Geometry: final body of the model. Coordinates: model frame, mm. A direction names the side the tool comes from. Coordinates: 2 decimals unless noted, no trailing zeros. Write each loop counter-clockwise with the first axis right and the second up, starting at its lowest first coordinate (ties: lowest second). Pieces come first, ordered by that corner, then holes.
Autodesk Inventor part; units mm, degrees
ref_plane "YZ Plane" through (0, 0, 0) normal (1, 0, 0) x (0, 1, 0)
ref_plane "XZ Plane" through (0, 0, 0) normal (0, 1, 0) x (-1, 0, 0)
ref_plane "XY Plane" through (0, 0, 0) normal (0, 0, 1) x (1, 0, 0)
sketch "Sketch1" plane through (0, 0, 0) normal (0, 0, 1) x (1, 0, 0)
  circle A0 centre (19.05, 19.05) radius 7.9375
  line L0 (22.7162, 25.4) -> (26.3823, 19.05)
  line L1 (26.3823, 19.05) -> (22.7162, 12.7)
  line L2 (22.7162, 12.7) -> (15.3838, 12.7)
  line L3 (15.3838, 12.7) -> (11.7177, 19.05)
  line L4 (11.7177, 19.05) -> (15.3838, 25.4)
  line L5 (15.3838, 25.4) -> (22.7162, 25.4)
  circle A1 centre (0, 19.05) radius 2.0828
  line L6 (0, 19.05) -> (19.05, 19.05) construction
  circle A2 centre (9.525, 2.5522) radius 2.0828
  circle A3 centre (28.575, 2.5522) radius 2.0828
  circle A4 centre (38.1, 19.05) radius 2.0828
  circle A5 centre (28.575, 35.5478) radius 2.0828
  circle A6 centre (9.525, 35.5478) radius 2.0828
  circle A7 centre (19.05, 19.05) radius 25.4
  line L7 (19.05, -6.35) -> (-19.05, -6.35)
  line L8 (-19.05, -6.35) -> (-19.05, 57.15)
  line L9 (6.3948, 114.3) -> (92.075, 114.3)
  line L10 (92.075, 114.3) -> (92.075, 63.5)
  line L11 (92.075, 63.5) -> (29.3317, 63.5)
  line L12 (-121.3454, 55.7276) -> (199.3502, 55.7276) construction
  arc A8 (29.3317, 63.5) -> (26.369, 43.3727) centre (29.3317, 53.2183) ccw
  circle A9 centre (85.725, 69.85) radius 2.0828
  circle A10 centre (85.725, 82.55) radius 2.0828
  circle A11 centre (85.725, 95.25) radius 2.0828
  circle A12 centre (85.725, 107.95) radius 2.0828
  line L13 (29.3317, 53.2183) -> (19.05, 53.2183) construction
  line L14 (-19.05, 57.15) -> (6.3948, 114.3)
  circle A13 centre (-12.7, 47.625) radius 2.0828
  circle A14 centre (6.35, 47.625) radius 2.0828
  circle A15 centre (-12.7, 22.225) radius 2.0828
  circle A16 centre (12.7, 78.7335) radius 2.0828
  circle A17 centre (12.7, 100.9585) radius 2.0828
  point P0 (0, 0)
  point P1 (19.05, 44.45)
  dimension "d7" = 15.875
  dimension "d8" = 12.7
  dimension "d23" = 4.1656
  dimension "d25" = 19.05
  dimension "d26" = 0
  dimension "d29" = 360
  dimension "d41" = 50.8
  dimension "d42" = 19.05
  dimension "d43" = 19.05
  dimension "d44" = 38.1
  dimension "d55" = 73.025
  dimension "d57" = 4.1656
  dimension "d58" = 6.35
  dimension "d59" = 6.35
  dimension "d62" = 12.7
  dimension "d67" = 6.35
  dimension "d68" = 36.6776
  dimension "d69" = 50.8
  dimension "d70" = 38.1
  dimension "d71" = 114
  dimension "d72" = 57.15
  dimension "d76" = 56.3933
  dimension "d78" = 6.35
  dimension "d79" = 9.525
  dimension "d84" = 19.05
  dimension "d91" = 31.75
  dimension "d98" = 25.4
  dimension "d105" = 22.225
  dimension "d113" = 6.35
extrude "Extrusion1" add sketch "Sketch1" along normal blind 3.175 contours A0 | A7 | A7 L7 L8 L14 L9 L10 L11 A8
sketch "Sketch2" plane through (0, 0, 3.175) normal (0, 0, 1) x (1, 0, 0)
  line L0 (-19.05, -6.35) -> (19.05, -6.35)
  arc A0 (19.05, -6.35) -> (26.369, 43.3727) centre (19.05, 19.05) ccw
  line L1 (-19.05, 57.15) -> (-19.05, -6.35)
  circle A1 centre (19.05, 19.05) radius 25.4
  line L2 (2.1167, 0.118) -> (-19.05, 19.05)
  line L3 (-19.05, 19.05) -> (-19.05, -6.35)
  line L4 (-19.05, -6.35) -> (19.05, -6.35)
  arc A2 (2.1167, 0.118) -> (19.05, -6.35) centre (19.05, 19.05) ccw
  point P0 (-19.05, 56.4751)
  point P1 (0, 0)
  dimension "d110" = 25.4
extrude "Extrusion2" cut sketch "Sketch2" against normal blind 25.4 contours L1 L2 A1 L0
fillet "Fillet2" radius 3.175 5 edges at (6.3948, 114.3, 1.5875) (-19.05, 57.15, 1.5875) (-19.05, 19.05, 1.5875) (92.075, 63.5, 1.5875) (92.075, 114.3, 1.5875)
equation "\"d67\" = d58"
properties part number "Lexan flexible Arm Mount" material "Polycarbonate, Clear"
Item 1: Section C-C, the plane x = -12.7. Output: boundary loops of the cut face in (y, z) (3 decimals).
Derived:
outline: (13.37, 0) - (20.142, 0) - (20.142, 3.175) - (13.37, 3.175) - close; (24.308, 0) - (45.542, 0) - (45.542, 3.175) - (24.308, 3.175) - close; (49.708, 0) - (71.412, 0) - (71.412, 3.175) - (49.708, 3.175) - close
Item 2: Section A-A, the plane x = 42.5. Output: boundary loops of the cut face in (y, z) (3 decimals).
Derived:
outline: (9.29, 0) - (28.81, 0) - (28.81, 3.175) - (9.29, 3.175) - close; (63.5, 0) - (114.3, 0) - (114.3, 3.175) - (63.5, 3.175) - close
Item 3: Pull-direction query (X, two-part tool) for faces 4 (the flat face through (92.075, 89, 2)), 5 (the cylindrical face through (85.273, 97.283, 1.565)), 6 (the cylindrical face through (6.75, 113.8, 1.61)); classes: released by +X, released by -X, zero draft, split by the parting line, or undercut.
Derived:
face 4: released by +X
face 5: undercut
face 6: released by -X
Item 4: Section D-D, the plane z = 2.6. State how many separate pieces and enclosed holes the cut face has, plus the area to 3 significant figures.
Derived:
separate pieces: 1
enclosed holes: 16
area: 7,910 mm2
Item 5: Section B-B, the plane y = 82.55. Output: boundary loops of the cut face in (x, z) (3 decimals), plus the area to 3 significant figures.
Derived:
outline: (-7.741, 0) - (83.642, 0) - (83.642, 3.175) - (-7.741, 3.175) - close; (87.808, 0) - (92.075, 0) - (92.075, 3.175) - (87.808, 3.175) - close
area: 304 mm2
Item 6: Set-up query: faces 1 (the flat face through (19, 12.7, 2)), 2 (the flat face through (-7.797, 8.985, 1.61)), 3 (the flat face through (60, 63.5, 2)). Return all of +Z, -Z, +X, -X, +Y, -Y with unobstructed straight access to the full face (end or side cutting, diameter ignored); none if empty.
Derived:
face 1: +Z, -Z
face 2: +Z, -Z, -X, -Y
face 3: +Z, -Z, +X
Item 7: Material intervals for probe 1 along Y at (x, z) = (-12.7, 1.25); probe 2 along X at (y, z) = (49, 2); probe 3 along Y at (x, z) = (14.5, 2.4), sorted ascending.
Derived:
probe 1: y = 13.37 to 20.14, 24.31 to 45.54, 49.71 to 71.41
probe 2: x = -19.05 to -14.26, -11.14 to 4.79, 7.91 to 19.96
probe 3: y = -5.94 to 14.23, 23.87 to 77.69, 79.78 to 99.91, 102.01 to 114.3
Item 8: Pin query (flat end, axial travel): pin 1 (2.5 mm diameter, centred on x = 12.7, y = 100.96, fed in from -Z); pin 2 (1 mm diameter, centred on y = 57.5, z = 0.5, fed in from +X); pin 3 (1.6 mm diameter, centred on x = 70, z = 1, fed in from -Y); pin 4 (1 mm diameter, centred on x = 20, z = 1.5, fed in from -Y). Return the tip coordinate at first contact, or that it passes through.
Derived:
pin 1: passes through
pin 2: stops at x = 20.23
pin 3: stops at y = 63.5
pin 4: stops at y = -6.35
